Source: CAD feature listing. Evaluate the final solid. Frame: model axes, mm. Round coordinates to 2 decimals unless told otherwise and drop trailing zeros. Loops run counter-clockwise (first coordinate to the right, second up) from the corner with the lowest first, then second, coordinate; pieces in that order, holes last. Notation, with made-up numbers: (30.5, 35.5) -> (57.5, 35.5) arc R21 cw to (57.5, 54.5) -> close; hole circle Ø5 at (7, 19.5). An arc over 180 degrees is marked (long way). Put each result on its own line as item: value. Start each with the question number.
1. Contact query for flat-ended pins moving along their axis: pin 1 (1.5 mm diameter, centred on x = -4, y = 310.5, fed in from +Z); pin 2 (1.5 mm diameter, centred on x = 0, z = 3.5, fed in from +Y); pin 3 (3 mm diameter, centred on x = -1, y = 170, fed in from -Z); pin 4 (12 mm diameter, centred on x = -3.5, y = 277.5, fed in from +Z). Output: stop coordinate, or through.
2. Cut plane A-A (y = 40.5). Return the cut outline in (x, z).
3. Material intervals for L1, parallel to Y at x = 8.45, z = 0 (3 decimals); L2, parallel to Y at x = 2.5, z = -4.25; L3, parallel to X at y = 260, z = 0.25, sorted ascending.
```python
from build123d import *

# Parameters (mm, degrees)
SKETCH1_R                     = 5.525
CORK_STOPPER_VACUMMPUMP_DEPTH = 10
SKETCH3_R                     = 2
LONGTHINSHAFT_DEPTH           = 400
SKETCH4_W                     = 20
SKETCH4_H                     = 15
BOSS_EXTRUDE3_DEPTH           = 32
CUT_EXTRUDE2_REACH            = 444.367
SKETCH5_W                     = 10
SKETCH5_H                     = 16
SKETCH7_R                     = 2.125
CUT_EXTRUDE3_DEPTH            = 20
FILLET1_R                     = 2
FILLET2_R                     = 2
FILLET3_R                     = 2


with BuildPart() as part:
    # Sketch1 → Cork/Stopper/VacummPump (new body)
    with BuildSketch(Plane(origin=(0, 0, 0), x_dir=(1, 0, 0), z_dir=(0, 1, 0))):
        with Locations(Location((0, 0, 0), (0, 0, 270))):
            Circle(SKETCH1_R)
    extrude(amount=CORK_STOPPER_VACUMMPUMP_DEPTH)

    # Sketch3 → LongThinShaft (add)
    with BuildSketch(Plane(origin=(0, 10, 0), x_dir=(1, 0, 0), z_dir=(0, 1, 0))):
        with Locations(Location((0, 0, 0), (0, 0, 270))):
            Circle(SKETCH3_R)
    extrude(amount=LONGTHINSHAFT_DEPTH)

    # Sketch4 → Boss-Extrude3 (add)
    with BuildSketch(Plane(origin=(0, 410, 0), x_dir=(1, 0, 0), z_dir=(0, 1, 0))):
        Rectangle(SKETCH4_W, SKETCH4_H)
    extrude(amount=BOSS_EXTRUDE3_DEPTH)

    # Sketch5 → Cut-Extrude2 (cut, up to next)
    with BuildSketch(Plane.XY.offset(7.5), mode=Mode.PRIVATE) as cut_extrude2_sk1:
        with Locations((0, 434)):
            Rectangle(SKETCH5_W, SKETCH5_H)
    cut_extrude2_tool1 = extrude(cut_extrude2_sk1.sketch, amount=-CUT_EXTRUDE2_REACH, mode=Mode.PRIVATE) & part.part
    add(cut_extrude2_tool1.solids().sort_by_distance((0, 434, 7.5))[0], mode=Mode.SUBTRACT)

    # Sketch7 → Cut-Extrude3 (cut)
    with BuildSketch(Plane.ZY.offset(10)):
        with Locations((0, 437.5)):
            Circle(SKETCH7_R)
    extrude(amount=-CUT_EXTRUDE3_DEPTH, mode=Mode.SUBTRACT)

    # Fillet1
    fillet1_edges = [part.edges().sort_by_distance(p)[0] for p in [
        (0, 410, -2),
    ]]
    fillet(fillet1_edges, radius=FILLET1_R)

    # Fillet2
    fillet2_edges = [part.edges().sort_by_distance(p)[0] for p in [
        (10, 410, 0),
        (10, 426, 7.5),
        (0, 410, -7.5),
        (10, 426, -7.5),
        (-10, 410, 0),
        (-10, 426, -7.5),
        (0, 410, 7.5),
        (-10, 426, 7.5),
        (10, 442, 0),
        (7.5, 442, -7.5),
        (-10, 442, 0),
        (-7.5, 442, 7.5),
        (-7.5, 442, -7.5),
        (7.5, 442, 7.5),
        (-5, 442, 0),
        (5, 434, -7.5),
        (5, 442, 0),
        (5, 434, 7.5),
        (-5, 434, 7.5),
        (0, 426, 7.5),
        (0, 426, -7.5),
        (-5, 434, -7.5),
    ]]
    fillet(fillet2_edges, radius=FILLET2_R)

    # Fillet3
    fillet3_edges = [part.edges().sort_by_distance(p)[0] for p in [
        (0, 10, -2),
    ]]
    fillet(fillet3_edges, radius=FILLET3_R)


solid = part.part
```
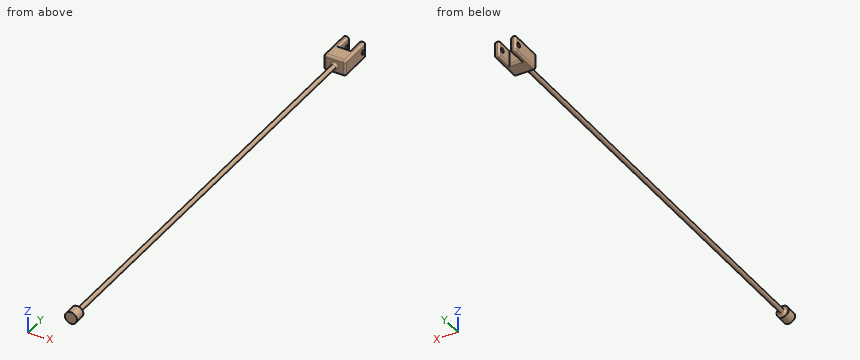
Solution:
1. pin 1: passes through
1. pin 2: stops at y = 426
1. pin 3: stops at z = -2
1. pin 4: stops at z = 2
2. outline: circle Ø4 at (0, 0)
3. L1: y = 410.051 to 435.375, 439.625 to 441.949
3. L2: y = 0 to 10, 410 to 426
3. L3: x = -1.98 to 1.98
